Geometry: final body of the model. Coordinates: model frame, mm. Face numbers are marked on the shaded views. Give positions to 0.01 mm unless a question says otherwise; leave off trailing zeros. Order: outer loops, then holes, each group sorted by start corner. A loop starts at its lowest first (then second) coordinate and runs counter-clockwise, first axis right, second up. Notation, with made-up numbers: (-18.75, 17) - (6.25, 17) arc R19 ccw to (6.25, 38) - close; hole circle Ø6 at (69, 6.25). An arc over 180 degrees is marked (long way). One line per item, written item: value.
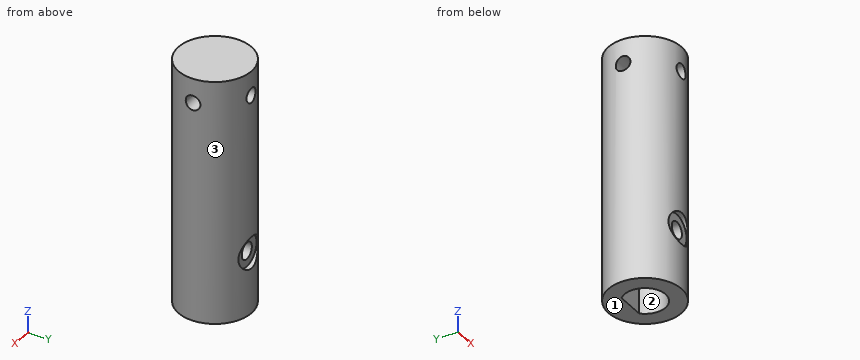
Autodesk Inventor part; units mm, degrees
ref_plane "作業平面1" through (7.5, 0, 0) normal (1, 0, 0) x (0, 1, 0)
ref_plane "作業平面2" through (-7.5, 0, 0) normal (1, 0, 0) x (0, 1, 0)
ref_plane "作業平面3" through (0, 7.5, 0) normal (0, 1, 0) x (-1, 0, 0)
sketch "スケッチ1" plane through (0, 0, 0) normal (0, 0, 1) x (1, 0, 0)
  circle A0 centre (0, 0) radius 7.5
  dimension "d0" = 15
extrude "押し出し1" add sketch "スケッチ1" along normal blind 50
sketch "スケッチ2" plane through (0, 0, 0) normal (0, 0, -1) x (-1, 0, 0)
  arc A0 (-2.9394, 3) -> (2.9394, 3) centre (0, 0) ccw
  line L0 (-2.9394, 3) -> (2.9394, 3)
  point P0 (-3.1305, 2.8)
  dimension "d3" = 4.2
  dimension "d4" = 3
extrude "押し出し2" cut sketch "スケッチ2" against normal blind 30
ref_plane "作業平面1" through (7.5, 0, 0) normal (1, 0, 0) x (0, 1, 0)
ref_plane "作業平面2" through (-7.5, 0, 0) normal (1, 0, 0) x (0, 1, 0)
ref_plane "作業平面3" through (0, 7.5, 0) normal (0, 1, 0) x (-1, 0, 0)
ref_plane "作業平面4" through (0, -7.5, 0) normal (0, 1, 0) x (-1, 0, 0)
sketch "スケッチ3" plane through (7.5, 0, 0) normal (1, 0, 0) x (0, 1, 0)
  circle A0 centre (0, 45) radius 1.5
  line L0 (7.5, 50) -> (-7.5, 50)
  point P0 (0, 0)
  dimension "d11" = 3
  dimension "d12" = 5
sketch "スケッチ4" plane through (-7.5, 0, 0) normal (1, 0, 0) x (0, 1, 0)
  circle A0 centre (0, 45) radius 1.5
  line L0 (7.5, 50) -> (-7.5, 50)
  point P0 (0, 0)
  dimension "d13" = 3
  dimension "d14" = 5
extrude "押し出し3" cut sketch "スケッチ3" against normal blind 5
extrude "押し出し4" cut sketch "スケッチ4" along normal blind 5
sketch "スケッチ5" plane through (0, 7.5, 0) normal (0, 1, 0) x (-1, 0, 0)
  circle A0 centre (0, 45) radius 1.5
  line L0 (7.5, 50) -> (-7.5, 50)
  point P0 (0, 0)
  dimension "d19" = 3
  dimension "d20" = 5
sketch "スケッチ6" plane through (0, -7.5, 0) normal (0, 1, 0) x (-1, 0, 0)
  circle A0 centre (0, 45) radius 1.5
  line L0 (7.5, 50) -> (-7.5, 50)
  point P0 (0, 0)
  dimension "d21" = 3
  dimension "d22" = 5
extrude "押し出し5" cut sketch "スケッチ5" against normal blind 5
extrude "押し出し6" cut sketch "スケッチ6" along normal blind 5
thread "ねじ1"
thread "ねじ2"
thread "ねじ3"
thread "ねじ4"
sketch "スケッチ7" plane through (0, 7.5, 0) normal (0, 1, 0) x (-1, 0, 0)
  circle A0 centre (0, 12.5) radius 1.7
  point P0 (0, 0)
  dimension "d35" = 3.4
  dimension "d36" = 12.5
extrude "押し出し7" cut sketch "スケッチ7" against normal through all
sketch "スケッチ8" plane through (0, 7.5, 0) normal (0, 1, 0) x (-1, 0, 0)
  circle A0 centre (0, 12.5) radius 3.25
  point P0 (0, 0)
  dimension "d39" = 6.5
  dimension "d40" = 12.5
sketch "スケッチ9" plane through (0, -7.5, 0) normal (0, 1, 0) x (-1, 0, 0)
  circle A0 centre (0, 12.5) radius 3.25
  point P0 (0, 0)
  dimension "d41" = 6.5
  dimension "d42" = 12.5
extrude "押し出し8" cut sketch "スケッチ8" against normal blind 1
extrude "押し出し9" cut sketch "スケッチ9" along normal blind 1
properties part number "rotary_transfer_shaft_5" material "ステンレス鋼"
1) Material intervals for line 1 along Z through (x, y) = (0, -6.7); line 2 along Z through (x, y) = (0, -5.9); line 3 along Y through (x, z) = (0, 5), sorted ascending.
Answers below:
line 1: 0 to 9.25, 15.75 to 43.5, 46.5 to 50
line 2: 0 to 10.8, 14.2 to 43.5, 46.5 to 50
line 3: -7.5 to -4.2, 3 to 7.5
2) Section A-A, the plane x = 0. Count the separate pieces of the cut face and the enclosed holes in it, then the cut area to 3 significant figures.
Answers below:
separate pieces: 3
enclosed holes: 0
area: 471 mm^2
3) Section B-B, the plane y = 0. Return loops of the section in (x, z), then the cut area to 3 significant figures.
Answers below:
outline: (-7.5, 0) - (-4.2, 0) - (-4.2, 30) - (4.2, 30) - (4.2, 0) - (7.5, 0) - (7.5, 43.5) - (2.5, 43.5) - (2.5, 46.5) - (7.5, 46.5) - (7.5, 50) - (-7.5, 50) - (-7.5, 46.5) - (-2.5, 46.5) - (-2.5, 43.5) - (-7.5, 43.5) - close
area: 468 mm^2
4) Mould query, pull axis Y, two halves, no side actions, for the marked faces 1, 2 and 3. Classes: released by +Y, released by -Y, zero draft, split by the parting line, or undercut.
Answers below:
face 1: zero draft
face 2: undercut
face 3: split by the parting line
5) Section D-D, the plane y = 4.5. Return loops of the section in (x, z), then the cut area to 3 significant figures.
Answers below:
outline: (-6, 0) - (6, 0) - (6, 50) - (-6, 50) - close; hole circle Ø3.4 at (0, 12.5); hole circle Ø3 at (0, 45)
area: 584 mm^2
6) Section C-C, the plane z = 24.5. Return loops of the section in (x, y).
Answers below:
outline: circle Ø15 at (0, 0); hole (-2.94, 3) arc R4.2 ccw (long way) to (2.94, 3) - close
7) First-contact query: pin 1 (8 mm diameter, centred on x = 4.5, z = 12.5, fed in from -Y); pin 2 (2.5 mm diameter, centred on y = 0, z = 45, fed in from +X); pin 3 (1 mm diameter, centred on x = 3, z = 12.5, fed in from +Y); pin 4 (2 mm diameter, centred on x = 0, z = 12.5, fed in from +Y). Flat tips, straight axial feed; report the tip coordinate or a pass-through.
Answers below:
pin 1: y = -7.32
pin 2: x = 2.5
pin 3: y = 6.77
pin 4: through
